```python
from build123d import *

# Parameters (mm, degrees)
SKETCH1_R           = 2
BOSS_EXTRUDE1_DEPTH = 4
FILLET1_R           = 3


with BuildPart() as part:
    # Sketch1 → Boss-Extrude1 (new body)
    with BuildSketch(Plane(origin=(0, 0, 0), x_dir=(1, 0, 0), z_dir=(0, 1, 0))):
        Polygon((0, 0), (20, 0), (20, 30), (30, 30), (30, 50), (0, 50), align=None)
        with Locations((10, 18.773227759)):
            Circle(SKETCH1_R, mode=Mode.SUBTRACT)
        with Locations((10, 8.773227759)):
            Circle(SKETCH1_R, mode=Mode.SUBTRACT)
        with Locations((20, 40)):
            Circle(SKETCH1_R, mode=Mode.SUBTRACT)
        with Locations((10, 40)):
            Circle(SKETCH1_R, mode=Mode.SUBTRACT)
    extrude(amount=BOSS_EXTRUDE1_DEPTH)

    # Fillet1
    fillet1_edges = [part.edges().sort_by_distance(p)[0] for p in [
        (0, 2, -50),
        (30, 2, -50),
        (30, 2, -30),
        (20, 2, -30),
        (20, 2, 0),
        (0, 2, 0),
    ]]
    fillet(fillet1_edges, radius=FILLET1_R)


solid = part.part
```
Model file for the job. Use its own axes, mm. A direction names the side the tool comes from. Coordinates: 2 decimals unless noted, no trailing zeros. Order: outer loops, then holes, each group sorted by start corner. A loop starts at its lowest first (then second) coordinate and runs counter-clockwise, first axis right, second up. Notation, with made-up numbers: (59, 8.5) - (100, 8.5) arc R20 ccw to (100, 44.5) - close; hole circle Ø1 at (-13.5, 43.5). An arc over 180 degrees is marked (long way). Return JSON: item names as keys, results as strings. Group by question number.
1) Saw through at C-C, the plane z = -9.5. Write the cut outline in (x, y).
2) Mould opens along Z. For faces 3 (the cylindrical face through (29.1, 2.03, -49.14)), 4 (the flat face through (11, 4, -31)), 5 (the cylindrical face through (9.74, 1.972, -20.756)) say: released by +Z, released by -Z, zero draft, split by the parting line, or undercut.
3) Flat gauge pins, fed straight in: P1, Ø3, axis at x = 20, z = -40, coming from the -Y side; P2, Ø1.2, axis at y = 2.5, z = -17.5, coming from the +X side. Where does each tip first touch, or does it go through?
4) Probe line 1 (X direction, y = 1, z = -40); line 2 (Z direction, x = 10, y = 3.05); line 3 (X direction, y = 3.3, z = -19). List the from-to ranges inside material, lowest first. Write a range as from..to.
5) Saw through at A-A, the plane z = -40. Write the cut outline in (x, y), plus the area to 3 significant figures.
6) Tool access for faces 1 (the flat face through (20, 2, -15)), 2 (the flat face through (11, 0, -31)): list every direction of +Z, -Z, +X, -X, +Y, -Y with a clear straight run to the whole face (end or side of a thin tool).
7) Saw through at D-D, the plane x = 18.5. Write the cut outline in (y, z), plus the area to 3 significant figures.
8) Saw through at B-B, the plane x = 10. Write the cut outline in (y, z).
Values found:
{
 "1": {"outline": "(0, 0) - (8.14, 0) - (8.14, 4) - (0, 4) - close; (11.86, 0) - (20, 0) - (20, 4) - (11.86, 4) - close"},
 "2": {"face 3": "released by -Z", "face 4": "zero draft", "face 5": "undercut"},
 "3": {"P1": "passes through", "P2": "stops at x = 20"},
 "4": {"line 1": "x = 0..8, 12..18, 22..30", "line 2": "z = -50..-42, -38..-20.77, -16.77..-10.77, -6.77..0", "line 3": "x = 0..8.01, 11.99..20"},
 "5": {"outline": "(0, 0) - (8, 0) - (8, 4) - (0, 4) - close; (12, 0) - (18, 0) - (18, 4) - (12, 4) - close; (22, 0) - (30, 0) - (30, 4) - (22, 4) - close", "area": "88.0 mm²"},
 "6": {"face 1": "+Z, +X, +Y, -Y", "face 2": "+Z, -Z, +X, -X, -Y"},
 "7": {"outline": "(0, -50) - (4, -50) - (4, -41.32) - (0, -41.32) - close; (0, -38.68) - (4, -38.68) - (4, -0.4) - (0, -0.4) - close", "area": "188 mm²"},
 "8": {"outline": "(0, -50) - (4, -50) - (4, -42) - (0, -42) - close; (0, -38) - (4, -38) - (4, -20.77) - (0, -20.77) - close; (0, -16.77) - (4, -16.77) - (4, -10.77) - (0, -10.77) - close; (0, -6.77) - (4, -6.77) - (4, 0) - (0, 0) - close"}
}
